from build123d import *

# Parameters (mm, degrees)
SKETCH1_W           = 18
SKETCH1_H           = 12
BOSS_EXTRUDE1_DEPTH = 4
BOSS_EXTRUDE2_DEPTH = 3
SKETCH3_R           = 1.75
CUT_EXTRUDE1_DEPTH  = 13.369316877
SKETCH4_R           = 4
CUT_EXTRUDE2_DEPTH  = 2.5
FILLET1_R           = 2


with BuildPart() as part:
    # Sketch1 → Boss-Extrude1 (new body)
    with BuildSketch(Plane.XY):
        Rectangle(SKETCH1_W, SKETCH1_H)
    extrude(amount=BOSS_EXTRUDE1_DEPTH)

    # Sketch2 → Boss-Extrude2 (add)
    with BuildSketch(Plane(origin=(9, 0, 0), x_dir=(0, 0, -1), z_dir=(1, 0, 0))):
        Polygon((-4, 6), (-10, 6), (-10, -6), (-4, -6), (-4, -3), (-7, -3), (-7, 3), (-4, 3), align=None)
    boss_extrude2 = extrude(amount=-BOSS_EXTRUDE2_DEPTH)

    # Mirror1: Boss-Extrude2 across plane
    add(boss_extrude2.mirror(Plane(origin=(0, 0, 0), x_dir=(0, 0, 1), z_dir=(1, 0, 0))))

    # Sketch3 → Cut-Extrude1 (cut, through all)
    with BuildSketch(Plane.XY.offset(4)):
        Circle(SKETCH3_R)
    extrude(amount=-CUT_EXTRUDE1_DEPTH, mode=Mode.SUBTRACT)

    # Sketch4 → Cut-Extrude2 (cut)
    with BuildSketch(Plane.XY.offset(4)):
        Circle(SKETCH4_R)
    extrude(amount=-CUT_EXTRUDE2_DEPTH, mode=Mode.SUBTRACT)

    # Fillet1
    fillet1_edges = [part.edges().sort_by_distance(p)[0] for p in [
        (-9, 6, 5),
        (9, 6, 5),
        (9, -6, 5),
        (-9, -6, 5),
    ]]
    fillet(fillet1_edges, radius=FILLET1_R)


solid = part.part
Work out the finished part from the listing and answer in its coordinate system (mm). A direction names the side the tool comes from. Round coordinates to 2 decimals unless told otherwise and drop trailing zeros. Write each loop counter-clockwise with the first axis right and the second up, starting at its lowest first coordinate (ties: lowest second). Pieces come first, ordered by that corner, then holes. Notation, with made-up numbers: M -2,72.5 L 38,72.5 A21 ccw 38,76.5 Z; hole C 29.5,82.25 d4. An arc over 180 degrees is marked long. Use a Markdown table: item, result.
1) The part is cut by section A-A on z = 8.25. Give the vertices of the cut face in (x, y).
Taken from the geometry:
| item | result |
|---|---|
| outline | M -9,-4 A2 ccw -7,-6 L -6,-6 L -6,6 L -7,6 A2 ccw -9,4 Z; M 6,-6 L 7,-6 A2 ccw 9,-4 L 9,4 A2 ccw 7,6 L 6,6 Z |
2) The part is cut by section C-C on x = 0. Give the vertices of the cut face in (y, z).
Taken from the geometry:
| item | result |
|---|---|
| outline | M -6,0 L -1.75,0 L -1.75,1.5 L -4,1.5 L -4,4 L -6,4 Z; M 1.75,0 L 6,0 L 6,4 L 4,4 L 4,1.5 L 1.75,1.5 Z |
3) Consider line 1 (Z direction, x = -6.75, y = -0.5); line 2 (Y direction, x = 0, z = 0.5); line 3 (X direction, y = -0.5, z = 8.25). Determine where each line is inside the solid, lowest interval first. Write a range as [from, to].
Taken from the geometry:
| item | result |
|---|---|
| line 1 | z = [0, 4], [7, 10] |
| line 2 | y = [-6, -1.75], [1.75, 6] |
| line 3 | x = [-9, -6], [6, 9] |
4) The part is cut by section D-D on z = 4.25. Give the vertices of the cut face in (x, y).
Taken from the geometry:
| item | result |
|---|---|
| outline | M -9,-4 A2 ccw -7,-6 L -6,-6 L -6,-3 L -9,-3 Z; M -9,3 L -6,3 L -6,6 L -7,6 A2 ccw -9,4 Z; M 6,-6 L 7,-6 A2 ccw 9,-4 L 9,-3 L 6,-3 Z; M 6,3 L 9,3 L 9,4 A2 ccw 7,6 L 6,6 Z |
5) The part is cut by section B-B on y = 0. Give the vertices of the cut face in (x, z).
Taken from the geometry:
| item | result |
|---|---|
| outline | M -9,0 L -1.75,0 L -1.75,1.5 L -4,1.5 L -4,4 L -9,4 Z; M -9,7 L -6,7 L -6,10 L -9,10 Z; M 1.75,0 L 9,0 L 9,4 L 4,4 L 4,1.5 L 1.75,1.5 Z; M 6,7 L 9,7 L 9,10 L 6,10 Z |
6) Which of the six approach directions +Z, -Z, +X, -X, +Y, -Y give full straight-line access (tool end or side, diameter ignored) to faces 1 (the face through (6, 0, 8)), 2 (the face through (8, 3, 6)), 3 (the face through (2, -1, 1.5)), 4 (the face through (-9, 0, 3))?
Taken from the geometry:
| item | result |
|---|---|
| face 1 | +Z, +Y, -Y |
| face 2 | +X, -X |
| face 3 | +Z |
| face 4 | +Z, -Z, -X, +Y, -Y |
7) Determine the mould class of faces 5 (the face through (2, 4, 4)), 6 (the face through (-2, 0, 0)), 7 (the face through (9, 0, 3)) for opening direction Z: pulls with the +Z half, pulls with the -Z half, needs draft (parallel to the pull), parting line crosses it, or undercut.
Taken from the geometry:
| item | result |
|---|---|
| face 5 | undercut |
| face 6 | pulls with the -Z half |
| face 7 | needs draft |
8) Flat-ended cylindrical pins translate along their axes: pin 1 (1.5 mm diameter, centred on x = -7, y = 1.5, fed in from -Z); pin 2 (4 mm diameter, centred on x = -2, y = -2, fed in from +Z); pin 3 (3.5 mm diameter, centred on x = 0, y = 1.5, fed in from +Z). Find the tip coordinate at first contact, or state that the pin passes through.
Taken from the geometry:
| item | result |
|---|---|
| pin 1 | stops at z = 0 |
| pin 2 | stops at z = 4 |
| pin 3 | stops at z = 1.5 |
